from build123d import *

# Parameters (mm, degrees)
BOSS_EXTRUDE1_DEPTH = 7.5
FILLET1_R           = 10
SKETCH2_R           = 4.975
CUT_EXTRUDE1_DEPTH  = 7.5
CHAMFER1_SIZE       = 1.5


with BuildPart() as part:
    # Sketch1 → Boss-Extrude1 (new body)
    with BuildSketch(Plane(origin=(0, 0, 0), x_dir=(1, 0, 0), z_dir=(0, 1, 0))):
        Polygon((70, 0), (20, 0), (20, -20), (0, -20), (0, -70), (20, -70), (20, -90), (70, -90), (70, -70), (90, -70), (90, -20), (70, -20), align=None)
    extrude(amount=BOSS_EXTRUDE1_DEPTH)

    # Fillet1
    # the kernel refuses this fillet: 10 mm, written as the material it takes off along each edge
    with BuildSketch(Plane(origin=(-24.206145914, 7.5, 70), x_dir=(0, -1, 0), z_dir=(1, 0, 0)), Plane(origin=(20, 7.5, 70), x_dir=(0, -1, 0), z_dir=(0, 0, 1)), Plane(origin=(70, 7.5, 114.206145914), x_dir=(0, -1, 0), z_dir=(0, 0, -1)), Plane(origin=(70, 7.5, 70), x_dir=(0, -1, 0), z_dir=(1, 0, 0)), Plane(origin=(114.206145914, 7.5, 20), x_dir=(0, -1, 0), z_dir=(-1, 0, 0)), Plane(origin=(70, 7.5, 20), x_dir=(0, -1, 0), z_dir=(0, 0, -1)), Plane(origin=(20, 7.5, -24.206145914), x_dir=(0, -1, 0), z_dir=(0, 0, 1)), Plane(origin=(20, 7.5, 20), x_dir=(0, -1, 0), z_dir=(-1, 0, 0))) as fillet1_piece_1:
        with BuildLine():
            CenterArc((10, 9.682458366), FILLET1_R, 180, 75.522487814)
            Line((0, 9.682458366), (-0.2, 9.682458366))
            Line((-0.2, 9.682458366), (-0.2, 0))
            Line((-0.2, 0), (0, -0.2))
            ThreePointArc((0, -0.2), (3.75, -0.2), (7.45, -0.193649167))
            Line((7.45, -0.193649167), (7.5, 0))
        make_face()
    extrude(amount=44.206145914, mode=Mode.SUBTRACT)
    with BuildSketch(Plane(origin=(-4.206145914, 7.5, 90), x_dir=(0, -1, 0), z_dir=(1, 0, 0)), Plane(origin=(90, 7.5, 94.206145914), x_dir=(0, -1, 0), z_dir=(0, 0, -1)), Plane(origin=(94.206145914, 7.5, 0), x_dir=(0, -1, 0), z_dir=(-1, 0, 0)), Plane(origin=(0, 7.5, -4.206145914), x_dir=(0, -1, 0), z_dir=(0, 0, 1))) as fillet1_piece_2:
        with BuildLine():
            CenterArc((10, 9.682458366), FILLET1_R, 180, 75.522487814)
            Line((0, 9.682458366), (-0.2, 9.682458366))
            Line((-0.2, 9.682458366), (-0.2, 0))
            Line((-0.2, 0), (0, -0.2))
            ThreePointArc((0, -0.2), (3.75, -0.2), (7.45, -0.193649167))
            Line((7.45, -0.193649167), (7.5, 0))
        make_face()
    extrude(amount=98.412291828, mode=Mode.SUBTRACT)
    with BuildSketch(Plane(origin=(-24.206145914, 7.5, 70), x_dir=(0, -1, 0), z_dir=(1, 0, 0))) as fillet1_piece_3a_section:
        with BuildLine():
            CenterArc((10, 9.682458366), FILLET1_R, 180, 75.522487814)
            Line((0, 9.682458366), (-0.2, 9.682458366))
            Line((-0.2, 9.682458366), (-0.2, 0))
            Line((-0.2, 0), (0, -0.2))
            ThreePointArc((0, -0.2), (3.75, -0.2), (7.45, -0.193649167))
            Line((7.45, -0.193649167), (7.5, 0))
        make_face()
    fillet1_piece_3a = extrude(amount=68.412291828, mode=Mode.PRIVATE)
    fillet1_piece_3a = split(fillet1_piece_3a, bisect_by=Plane(origin=(20, 5.604082443, 67.718558992), z_dir=(1, 0, 0)), keep=Keep.TOP, mode=Mode.PRIVATE)
    with BuildSketch(Plane(origin=(20, 7.5, 45.793854086), x_dir=(0, -1, 0), z_dir=(0, 0, 1))) as fillet1_piece_3b_section:
        with BuildLine():
            CenterArc((10, 9.682458366), FILLET1_R, 180, 75.522487814)
            Line((0, 9.682458366), (-0.2, 9.682458366))
            Line((-0.2, 9.682458366), (-0.2, 0))
            Line((-0.2, 0), (0, -0.2))
            ThreePointArc((0, -0.2), (3.75, -0.2), (7.45, -0.193649167))
            Line((7.45, -0.193649167), (7.5, 0))
        make_face()
    fillet1_piece_3b = extrude(amount=68.412291828, mode=Mode.PRIVATE)
    fillet1_piece_3b = split(fillet1_piece_3b, bisect_by=Plane(origin=(22.281441008, 5.604082443, 70), z_dir=(0, 0, -1)), keep=Keep.TOP, mode=Mode.PRIVATE)
    fillet1_piece_3 = fillet1_piece_3a & fillet1_piece_3b
    add(fillet1_piece_3, mode=Mode.SUBTRACT)
    with BuildSketch(Plane(origin=(70, 7.5, 114.206145914), x_dir=(0, -1, 0), z_dir=(0, 0, -1))) as fillet1_piece_4a_section:
        with BuildLine():
            CenterArc((10, 9.682458366), FILLET1_R, 180, 75.522487814)
            Line((0, 9.682458366), (-0.2, 9.682458366))
            Line((-0.2, 9.682458366), (-0.2, 0))
            Line((-0.2, 0), (0, -0.2))
            ThreePointArc((0, -0.2), (3.75, -0.2), (7.45, -0.193649167))
            Line((7.45, -0.193649167), (7.5, 0))
        make_face()
    fillet1_piece_4a = extrude(amount=68.412291828, mode=Mode.PRIVATE)
    fillet1_piece_4a = split(fillet1_piece_4a, bisect_by=Plane(origin=(67.718558992, 5.604082443, 70), z_dir=(0, 0, -1)), keep=Keep.TOP, mode=Mode.PRIVATE)
    with BuildSketch(Plane(origin=(45.793854086, 7.5, 70), x_dir=(0, -1, 0), z_dir=(1, 0, 0))) as fillet1_piece_4b_section:
        with BuildLine():
            CenterArc((10, 9.682458366), FILLET1_R, 180, 75.522487814)
            Line((0, 9.682458366), (-0.2, 9.682458366))
            Line((-0.2, 9.682458366), (-0.2, 0))
            Line((-0.2, 0), (0, -0.2))
            ThreePointArc((0, -0.2), (3.75, -0.2), (7.45, -0.193649167))
            Line((7.45, -0.193649167), (7.5, 0))
        make_face()
    fillet1_piece_4b = extrude(amount=68.412291828, mode=Mode.PRIVATE)
    fillet1_piece_4b = split(fillet1_piece_4b, bisect_by=Plane(origin=(70, 5.604082443, 67.718558992), z_dir=(-1, 0, 0)), keep=Keep.TOP, mode=Mode.PRIVATE)
    fillet1_piece_4 = fillet1_piece_4a & fillet1_piece_4b
    add(fillet1_piece_4, mode=Mode.SUBTRACT)
    with BuildSketch(Plane(origin=(114.206145914, 7.5, 20), x_dir=(0, -1, 0), z_dir=(-1, 0, 0))) as fillet1_piece_5a_section:
        with BuildLine():
            CenterArc((10, 9.682458366), FILLET1_R, 180, 75.522487814)
            Line((0, 9.682458366), (-0.2, 9.682458366))
            Line((-0.2, 9.682458366), (-0.2, 0))
            Line((-0.2, 0), (0, -0.2))
            ThreePointArc((0, -0.2), (3.75, -0.2), (7.45, -0.193649167))
            Line((7.45, -0.193649167), (7.5, 0))
        make_face()
    fillet1_piece_5a = extrude(amount=68.412291828, mode=Mode.PRIVATE)
    fillet1_piece_5a = split(fillet1_piece_5a, bisect_by=Plane(origin=(70, 5.604082443, 22.281441008), z_dir=(-1, 0, 0)), keep=Keep.TOP, mode=Mode.PRIVATE)
    with BuildSketch(Plane(origin=(70, 7.5, 44.206145914), x_dir=(0, -1, 0), z_dir=(0, 0, -1))) as fillet1_piece_5b_section:
        with BuildLine():
            CenterArc((10, 9.682458366), FILLET1_R, 180, 75.522487814)
            Line((0, 9.682458366), (-0.2, 9.682458366))
            Line((-0.2, 9.682458366), (-0.2, 0))
            Line((-0.2, 0), (0, -0.2))
            ThreePointArc((0, -0.2), (3.75, -0.2), (7.45, -0.193649167))
            Line((7.45, -0.193649167), (7.5, 0))
        make_face()
    fillet1_piece_5b = extrude(amount=68.412291828, mode=Mode.PRIVATE)
    fillet1_piece_5b = split(fillet1_piece_5b, bisect_by=Plane(origin=(67.718558992, 5.604082443, 20), z_dir=(0, 0, 1)), keep=Keep.TOP, mode=Mode.PRIVATE)
    fillet1_piece_5 = fillet1_piece_5a & fillet1_piece_5b
    add(fillet1_piece_5, mode=Mode.SUBTRACT)
    with BuildSketch(Plane(origin=(20, 7.5, -24.206145914), x_dir=(0, -1, 0), z_dir=(0, 0, 1))) as fillet1_piece_6a_section:
        with BuildLine():
            CenterArc((10, 9.682458366), FILLET1_R, 180, 75.522487814)
            Line((0, 9.682458366), (-0.2, 9.682458366))
            Line((-0.2, 9.682458366), (-0.2, 0))
            Line((-0.2, 0), (0, -0.2))
            ThreePointArc((0, -0.2), (3.75, -0.2), (7.45, -0.193649167))
            Line((7.45, -0.193649167), (7.5, 0))
        make_face()
    fillet1_piece_6a = extrude(amount=68.412291828, mode=Mode.PRIVATE)
    fillet1_piece_6a = split(fillet1_piece_6a, bisect_by=Plane(origin=(22.281441008, 5.604082443, 20), z_dir=(0, 0, 1)), keep=Keep.TOP, mode=Mode.PRIVATE)
    with BuildSketch(Plane(origin=(44.206145914, 7.5, 20), x_dir=(0, -1, 0), z_dir=(-1, 0, 0))) as fillet1_piece_6b_section:
        with BuildLine():
            CenterArc((10, 9.682458366), FILLET1_R, 180, 75.522487814)
            Line((0, 9.682458366), (-0.2, 9.682458366))
            Line((-0.2, 9.682458366), (-0.2, 0))
            Line((-0.2, 0), (0, -0.2))
            ThreePointArc((0, -0.2), (3.75, -0.2), (7.45, -0.193649167))
            Line((7.45, -0.193649167), (7.5, 0))
        make_face()
    fillet1_piece_6b = extrude(amount=68.412291828, mode=Mode.PRIVATE)
    fillet1_piece_6b = split(fillet1_piece_6b, bisect_by=Plane(origin=(20, 5.604082443, 22.281441008), z_dir=(1, 0, 0)), keep=Keep.TOP, mode=Mode.PRIVATE)
    fillet1_piece_6 = fillet1_piece_6a & fillet1_piece_6b
    add(fillet1_piece_6, mode=Mode.SUBTRACT)

    # Sketch2 → Cut-Extrude1 (cut)
    with BuildSketch(Plane(origin=(0, 7.5, 0), x_dir=(1, 0, 0), z_dir=(0, 1, 0))):
        with Locations(Location((45.317541634, -44.682458366, 0), (0, 0, 270))):
            Circle(SKETCH2_R)
    extrude(amount=-CUT_EXTRUDE1_DEPTH, mode=Mode.SUBTRACT)

    # Chamfer1
    chamfer1_edges = [part.edges().sort_by_distance(p)[0] for p in [
        (45.317541634, 0, 39.707458366),
    ]]
    chamfer(chamfer1_edges, length=CHAMFER1_SIZE)


solid = part.part
Source: CAD feature listing. Evaluate the final solid. Frame: model axes, mm. A direction names the side the tool comes from. Give positions to 0.01 mm unless a question says otherwise; leave off trailing zeros. Write each loop counter-clockwise with the first axis right and the second up, starting at its lowest first coordinate (ties: lowest second). Pieces come first, ordered by that corner, then holes. Notation, with made-up numbers: (-19.5, 31) -> (-10.5, 31) arc R18 ccw to (-10.5, 51) -> close; hole circle Ø11 at (7, -28). An arc over 180 degrees is marked (long way). Write item = value, one per line.
Q1. Reachability of faces 1 (the face through (23.63, 5.46, 74.95)), 2 (the face through (66.37, 5.46, 15.05)), 3 (the face through (23.63, 5.46, 14.63)) from +Z, -Z, +X, -X, +Y, -Y: full face, straight path, thin tool, end or side. Return the list, or none.
Here are the results:
face_1 = +Z, -X, +Y
face_2 = -Z, +X, +Y
face_3 = -Z, -X, +Y
Q2. Mould query, pull axis Z, two halves, no side actions, for faces 4 (the face through (42.29, 4.542, 40.734)), 5 (the face through (45, 7.5, 52)), 6 (the face through (45.35, 5.46, 3.63)), 7 (the face through (14.63, 5.46, 66.37)). Classes: +Z half, -Z half, draft (parallel to the pull), parting line (faces both ways), or undercut.
Here are the results:
face_4 = undercut
face_5 = draft
face_6 = -Z half
face_7 = +Z half
Q3. Cut plane B-B on x = 16. Return loops of the section in (y, z), then the cut area to 3 significant figures.
Here are the results:
outline = (0, 20) arc R10 ccw to (7.5, 29.68) -> (7.5, 60.32) arc R10 ccw to (0, 70) -> close
area = 337 mm²
Q4. Cut plane A-A on y = 3.75. Return loops of the section in (x, z) (3 decimals).
Here are the results:
outline = (1.876, 21.876) -> (21.876, 21.876) -> (21.876, 1.876) -> (68.124, 1.876) -> (68.124, 21.876) -> (88.124, 21.876) -> (88.124, 68.124) -> (68.124, 68.124) -> (68.124, 88.124) -> (21.876, 88.124) -> (21.876, 68.124) -> (1.876, 68.124) -> close; hole circle Ø9.95 at (45.318, 44.682)
Q5. Cut plane D-D on z = 66. Return loops of the section in (x, y), then the cut area to 3 significant figures.
Here are the results:
outline = (0, 0) -> (90, 0) arc R10 ccw to (86, 5.73) -> (66, 5.73) arc R10 ccw to (60.32, 7.5) -> (29.68, 7.5) arc R10 ccw to (24, 5.73) -> (4, 5.73) arc R10 ccw to start
area = 567 mm²
Q6. Cut plane C-C on z = 16. Return loops of the section in (x, y), then the cut area to 3 significant figures.
Here are the results:
outline = (20, 0) -> (70, 0) arc R10 ccw to (60.32, 7.5) -> (29.68, 7.5) arc R10 ccw to start
area = 337 mm²
Q7. First-contact query: pin 1 (11.5 mm diameter, centred on x = 45.32, z = 44.68, fed in from -Y); pin 2 (1 mm diameter, centred on y = 1.5, z = 17, fed in from -X); pin 3 (1 mm diameter, centred on y = 3.5, z = 43.5, fed in from +X). Flat tips, straight axial feed; report the tip coordinate or a pass-through.
Here are the results:
pin_1 = 0.72
pin_2 = 20.31
pin_3 = 88.67
Q8. Line query: line 1 (X direction, y = 4.75, z = 46.5); line 2 (Z direction, x = 85, y = 2.5); line 3 (Y direction, x = 27, z = 77). Output: solid intervals per line, ascending. Write a range as from..to.
Here are the results:
line_1 = 2.79..40.69, 49.95..87.21
line_2 = 21.02..68.98
line_3 = 0..7.13
